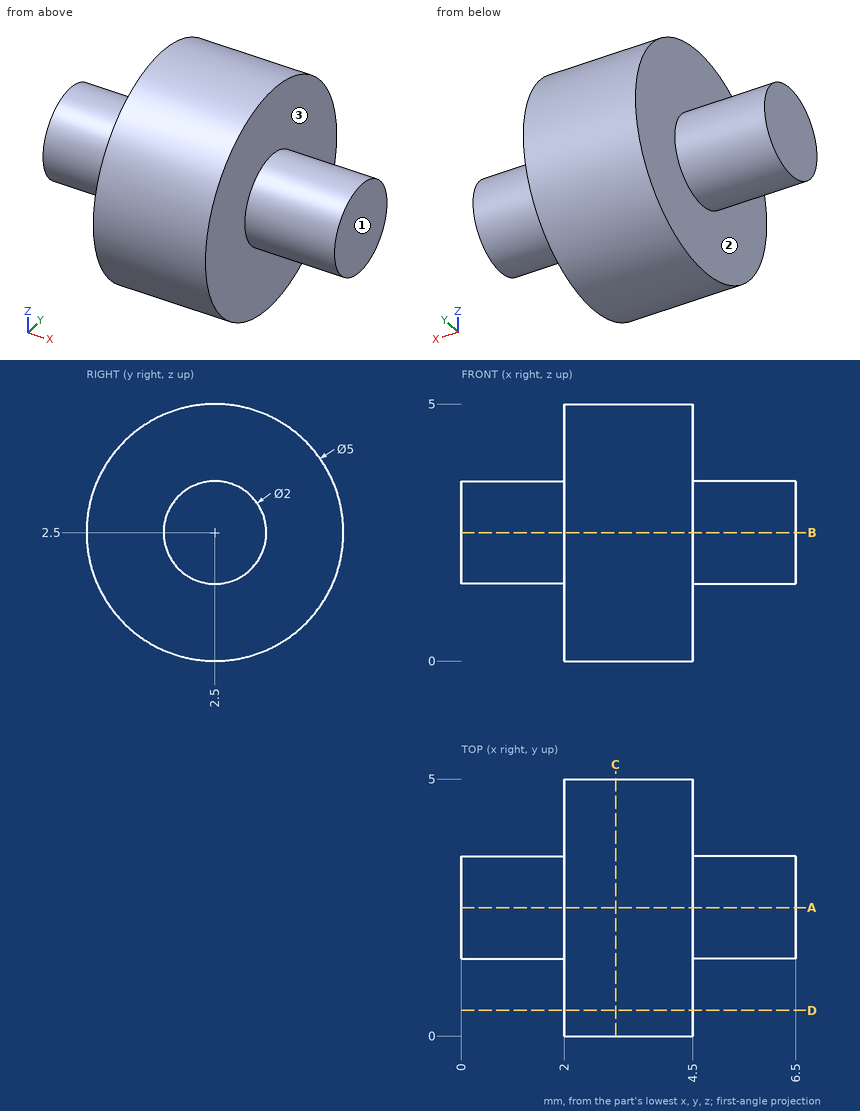
Here's the drawing with two shaded views (mm, measured from the low corner). I have some questions. A direction names the side the tool comes from. Coordinates: 2 decimals unless noted, no trailing zeros. Order: outer loops, then holes, each group sorted by start corner. A loop starts at its lowest first (then second) coordinate and runs counter-clockwise, first axis right, second up.
Item 1: If we section it at C-C on x = 3: List the corners of the cut face in (y, z) for me.
Result sheet:
outline: circle Ø5 at (2.5, 2.5)
Item 2: I need wall thicknesses on line 1 (X direction, y = 1.6, z = 1); line 2 (Z direction, x = 0.75, y = 2.45). Which ranges of each line are inside material? Lowest first, please.
Result sheet:
line 1: x = 2 to 4.5
line 2: z = 1.5 to 3.5
Item 3: If we section it at D-D on y = 0.5: List the corners of the cut face in (x, z) for me, plus the area to 3 significant figures.
Result sheet:
outline: (2, 1) - (4.5, 1) - (4.5, 4) - (2, 4) - close
area: 7.50 mm2
Item 4: For P1, Ø1.5, axis at y = 1, z = 2.5, coming from the -X side; P2, Ø1, axis at x = 2.5, z = 3.5, coming from the +Y side; P3, Ø1, axis at y = 1, z = 4.5, coming from the -X side, each with a flat end and sliding along its axis, tell me the tip position at first contact or that it passes through.
Result sheet:
P1: stops at x = 0
P2: stops at y = 4.95
P3: stops at x = 2
Item 5: If we section it at A-A on y = 2.5: List the corners of the cut face in (x, z) for me, plus the area to 3 significant figures.
Result sheet:
outline: (0, 1.5) - (2, 1.5) - (2, 0) - (4.5, 0) - (4.5, 1.5) - (6.5, 1.5) - (6.5, 3.5) - (4.5, 3.5) - (4.5, 5) - (2, 5) - (2, 3.5) - (0, 3.5) - close
area: 20.5 mm2
Item 6: For the marked faces 1, 2 and 3, which set-ups out of +Z, -Z, +X, -X, +Y, -Y let a thin tool reach every point of the face, with its end or its side?
Result sheet:
face 1: +Z, -Z, +X, +Y, -Y
face 2: -X
face 3: +X
